Work out the finished part from the listing and answer in its coordinate system (mm). A direction names the side the tool comes from. Give positions to 0.01 mm unless a question says otherwise; leave off trailing zeros. Write each loop counter-clockwise with the first axis right and the second up, starting at its lowest first coordinate (ties: lowest second). Pieces come first, ordered by that corner, then holes.
1) Straight lines are drawn through the part: probe 1 along Z at (x, y) = (-76.2, 4.75); probe 2 along X at (y, z) = (4.25, -57.15); probe 3 along X at (y, z) = (2.5, 12). For each, find the intervals that lie inside material, in ascending order.
2) Find section B-B (z = -13.5). Determine the outline of the cut face in (x, y) (3 decimals).
3) A tool of negligible diameter and unlimited length cuts with its end or side. For faces 4 (the face through (-82.55, 3, 1)), 5 (the face through (44, -3.175, 6)), from which of +Z, -Z, +X, -X, +Y, -Y can it reach the whole face along a straight path? Write none if from no direction.
4) Determine the mould class of faces 1 (the face through (-1, 3, 63.5)), 2 (the face through (-1, 6.35, -1)), 3 (the face through (-29, 3.175, 6)) for opening direction Z: pulls with the +Z half, pulls with the -Z half, needs draft (parallel to the pull), parting line crosses it, or undercut.
5) Find section C-C (z = -45.5). Determine the outline of the cut face in (x, y), plus the area to 3 significant figures.
6) Given pin 1 Ø4 at (x, z) = (0, 57.15) entering from +Y; pin 2 Ø3 at (x, z) = (-23.5, 0) entering from -Y (3 decimals); pin 3 Ø8 at (x, z) = (76.2, 0) entering from +Y; pin 4 Ø1 at (x, z) = (31, 31.5) entering from -Y, each flat-ended and moving along its own axis, determine where each tip first touches the part or whether it passes through.
7) Find section D-D (x = 62). Determine the outline of the cut face in (y, z).
```python
from build123d import *

# Parameters (mm, degrees)
SKETCH1_W                                        = 165.1
SKETCH1_H                                        = 127
SKETCH1_R                                        = 7.14375
SKETCH1_R_2                                      = 7.9375
BOSS_EXTRUDE1_DEPTH                              = 6.35
SKETCH2_R                                        = 28.575
SKETCH2_R_2                                      = 7.14375
SKETCH2_R_3                                      = 12.7
SKETCH2_R_4                                      = 7.9375
BOSS_EXTRUDE2_DEPTH                              = 15.875
SKETCH3_R                                        = 8.73125
CUT_EXTRUDE1_DEPTH                               = 3.175
SKETCH4_R                                        = 23.8125
CUT_EXTRUDE2_DEPTH                               = 12.7
BOSS_EXTRUDE4_START                              = 3.175
SKETCH5_R                                        = 7.9375
BOSS_EXTRUDE4_DEPTH                              = 6.35
CSK_FOR_1_4_FLAT_HEAD_MACHINE_SCREW1_D           = 6.7564
CSK_FOR_1_4_FLAT_HEAD_MACHINE_SCREW1_CSINK_D     = 12.8778
CSK_FOR_1_4_FLAT_HEAD_MACHINE_SCREW1_CSINK_ANGLE = 82
FILLET1_R                                        = 6.35
F_10_CLEARANCE_HOLE1_D                           = 5.1054


with BuildPart() as part:
    # Sketch1 → Boss-Extrude1 (new body)
    with BuildSketch(Plane(origin=(0, 0, 0), x_dir=(1, 0, 0), z_dir=(0, 1, 0))):
        Rectangle(SKETCH1_W, SKETCH1_H)
        with Locations((-19.05, -6.35)):
            Circle(SKETCH1_R, mode=Mode.SUBTRACT)
        with Locations((44.45, -6.35)):
            Circle(SKETCH1_R_2, mode=Mode.SUBTRACT)
    extrude(amount=BOSS_EXTRUDE1_DEPTH)

    # Sketch2 → Boss-Extrude2 (add)
    with BuildSketch(Plane(origin=(0, 6.35, 0), x_dir=(1, 0, 0), z_dir=(0, 1, 0))):
        with Locations((-19.05, -6.35)):
            Circle(SKETCH2_R)
        with Locations((-19.05, -6.35)):
            Circle(SKETCH2_R_2, mode=Mode.SUBTRACT)
        with Locations((44.45, -6.35)):
            Circle(SKETCH2_R_3)
        with Locations((44.45, -6.35)):
            Circle(SKETCH2_R_4, mode=Mode.SUBTRACT)
    extrude(amount=-BOSS_EXTRUDE2_DEPTH)

    # Sketch3 → Cut-Extrude1 (cut)
    with BuildSketch(Plane.XZ.offset(-6.35)):
        with Locations((-19.05, 6.35)):
            Circle(SKETCH3_R)
    extrude(amount=CUT_EXTRUDE1_DEPTH, mode=Mode.SUBTRACT)

    # Sketch4 → Cut-Extrude2 (cut)
    with BuildSketch(Plane(origin=(0, -9.525, 0), x_dir=(-1, 0, 0), z_dir=(0, -1, 0))):
        with Locations((19.05, -6.35)):
            Circle(SKETCH4_R)
    extrude(amount=-CUT_EXTRUDE2_DEPTH, mode=Mode.SUBTRACT)

    # Sketch5 → Boss-Extrude4 (add)
    with BuildSketch(Plane.XZ.offset(BOSS_EXTRUDE4_START)):
        with Locations((44.45, 6.35)):
            Circle(SKETCH5_R)
    extrude(amount=BOSS_EXTRUDE4_DEPTH)

    # CSK for 1/4 Flat Head Machine Screw1 (through all)
    with Locations(Plane(origin=(0, 6.35, 0), x_dir=(1, 0, 0), z_dir=(0, 1, 0))):
        with Locations((-61.255686472, -6.291233063), (15.015571308, 21.800289443), (-2.54, -43.18)):
            CounterSinkHole(CSK_FOR_1_4_FLAT_HEAD_MACHINE_SCREW1_D / 2, CSK_FOR_1_4_FLAT_HEAD_MACHINE_SCREW1_CSINK_D / 2, counter_sink_angle=CSK_FOR_1_4_FLAT_HEAD_MACHINE_SCREW1_CSINK_ANGLE)

    # Fillet1
    fillet1_edges = [part.edges().sort_by_distance(p)[0] for p in [
        (-82.55, 3.175, -63.5),
        (82.55, 3.175, -63.5),
        (82.55, 3.175, 63.5),
        (-82.55, 3.175, 63.5),
    ]]
    fillet(fillet1_edges, radius=FILLET1_R)

    # #10 Clearance Hole1 (through all)
    with Locations(Plane(origin=(0, 6.35, 0), x_dir=(1, 0, 0), z_dir=(0, 1, 0))):
        with Locations((-76.2, -57.15), (-76.2, 57.15), (76.2, 57.15), (76.2, -57.15), (0, 57.15), (0, -57.15), (-76.2, 0), (76.2, 0)):
            Hole(F_10_CLEARANCE_HOLE1_D / 2)


solid = part.part
```
Results:
1. probe 1: z = -63.5 to -59.7, -54.6 to -2.55, 2.55 to 54.6, 59.7 to 63.5
1. probe 2: x = -82.55 to -78.75, -73.65 to -2.55, 2.55 to 73.65, 78.75 to 82.55
1. probe 3: x = -82.55 to -42.18, 4.08 to 38.87, 50.03 to 82.55
2. outline: (-82.55, 0) - (-39.605, 0) - (-39.605, -9.525) - (-32.203, -9.525) - (-32.203, 3.175) - (-5.897, 3.175) - (-5.897, -9.525) - (1.505, -9.525) - (1.505, 0) - (82.55, 0) - (82.55, 6.35) - (-82.55, 6.35) - close
3. face 4: +Z, -Z, -X, +Y, -Y
3. face 5: +Y
4. face 1: pulls with the +Z half
4. face 2: needs draft
4. face 3: undercut
5. outline: (-82.55, 0) - (82.55, 0) - (82.55, 6.35) - (-82.55, 6.35) - close
5. area: 1,050 mm2
6. pin 1: passes through
6. pin 2: stops at y = 3.175
6. pin 3: stops at y = 6.35
6. pin 4: stops at y = 0
7. outline: (0, -63.5) - (6.35, -63.5) - (6.35, 63.5) - (0, 63.5) - close
